Geometry: final body of the model. Coordinates: model frame, mm. A direction names the side the tool comes from. Give positions to 0.01 mm unless a question says otherwise; leave off trailing zeros. Write each loop counter-clockwise with the first axis right and the second up, starting at its lowest first coordinate (ties: lowest second). Pieces come first, ordered by that corner, then holes. Notation, with made-up numbers: M -39.5,-5.75 L -23.5,-5.75 A22 ccw -23.5,7.25 Z; hole C 17.25,69.5 d2. An arc over 180 degrees is marked long. Use a Markdown table: item, result. Add a question column.
(1) Cut plane A-A (z = -4.5). Output: boundary loops of the cut face in (x, y).
(2) Pin query (flat end, axial travel): pin 1 Ø1 at (x, y) = (-1.5, -3.5) entering from -Z; pin 2 Ø1.5 at (y, z) = (-1, -3.5) entering from +X. Return the tip coordinate at first contact, or that it passes through.
(3) Material intervals for L1, parallel to X at y = -3.75, z = 4.75; L2, parallel to Z at x = -1, y = -2.25; L3, parallel to X at y = -3, z = -0.5, sorted ascending.
(4) Draft query along Z for faces 1 (the flat face through (-0.04, -2.99, -6.58)), 2 (the flat face through (0, 0, 0)), 3 (the conical face through (8.223, -1.972, 6.114)), 4 (the conical face through (-1.35, -3.288, 1.375)). Return one class per face: released by +Z, released by -Z, zero draft, split by the parting line, or undercut.
(5) Reachability of faces 5 (the flat face through (0.04, -2.99, 6.58)), 6 (the flat face through (0, -6, -2)), 7 (the conical face through (8.24, -1.97, -6.1)), 8 (the conical face through (-8.24, -1.97, 6.1)), 9 (the conical face through (1.375, -3.288, 1.35)) from +Z, -Z, +X, -X, +Y, -Y: full face, straight path, thin tool, end or side. Return the list, or none.
(6) Cut plane B-B (y = -1.75). State how many separate pieces and enclosed holes the cut face has, plus the area to 3 significant figures.
```python
from build123d import *

# Parameters (mm, degrees)
BOSS_EXTRUDE1_DEPTH = 4
BOSS_EXTRUDE1_DRAFT = 1
SHELL1_T            = -0.5
SKETCH2_R           = 2
BOSS_EXTRUDE2_DEPTH = 5.5
BOSS_EXTRUDE2_TAPER = 1.5
SKETCH4_R           = 1.605977431
CUT_EXTRUDE1_DEPTH  = 5.5
CUT_EXTRUDE1_DRAFT  = 1.5
BOSS_EXTRUDE3_DEPTH = 2.5
BOSS_EXTRUDE4_DEPTH = 2.5


with BuildPart() as part:
    # Sketch1 → Boss-Extrude1 (with draft: the straight prism first)
    with BuildSketch(Plane(origin=(0, 0, 0), x_dir=(1, 0, 0), z_dir=(0, 1, 0))):
        with BuildLine():
            Line((-7.5, -6.375), (7.5, -6.375))
            ThreePointArc((7.5, -6.375), (8.207106781, -6.082106781), (8.5, -5.375))
            Line((8.5, -5.375), (8.5, 5.375))
            ThreePointArc((8.5, 5.375), (8.207106781, 6.082106781), (7.5, 6.375))
            Line((7.5, 6.375), (-7.5, 6.375))
            ThreePointArc((-7.5, 6.375), (-8.207106781, 6.082106781), (-8.5, 5.375))
            Line((-8.5, 5.375), (-8.5, -5.375))
            ThreePointArc((-8.5, -5.375), (-8.207106781, -6.082106781), (-7.5, -6.375))
        make_face()
    extrude(amount=-BOSS_EXTRUDE1_DEPTH)
    # Boss-Extrude1: the draft: its side faces are tilted about the plane it starts from
    boss_extrude1_sides = [part.faces().sort_by_distance(p)[0] for p in [
        (0, -2, 6.375),
        (8.207106781, -2, 6.082106781),
        (8.5, -2, 0),
        (8.207106781, -2, -6.082106781),
        (0, -2, -6.375),
        (-8.207106781, -2, -6.082106781),
        (-8.5, -2, 0),
        (-8.207106781, -2, 6.082106781),
    ]]
    draft(boss_extrude1_sides, Plane(origin=(0, 0, 0), x_dir=(1, 0, 0), z_dir=(0, 1, 0)), BOSS_EXTRUDE1_DRAFT)

    # Shell1
    shell1_openings = [part.faces().sort_by_distance(p)[0] for p in [
        (0, -4, 0),
    ]]
    offset(amount=SHELL1_T, openings=shell1_openings, kind=Kind.INTERSECTION)

    # Sketch2 → Boss-Extrude2 (add)
    with BuildSketch(Plane.XZ.offset(0.5)):
        Circle(SKETCH2_R)
    extrude(amount=BOSS_EXTRUDE2_DEPTH, taper=BOSS_EXTRUDE2_TAPER)

    # Rib1: read off the stored shape, not the designer's step
    # Rib1: loft between two sections, ruled curve by curve
    rib1_from = [
        Edge.make_line((1.982008604, -0.5, 0.267660037), (3, -0.5, 0.25)),
        Edge.make_line((1.982008604, -0.5, -0.267660037), (3, -0.5, -0.25)),
        Edge.make_line((3, -0.5, -0.25), (3, -0.5, 0.25)),
        Edge.make_line((1.982008604, -0.5, -0.267660037), (1.982008604, -0.5, 0.267660037)),
    ]
    rib1_to = [
        Edge.make_line((1.83774048, -6, 0.259542201), (2.387789079, -6, 0.25)),
        Edge.make_line((1.83774048, -6, -0.259542201), (2.387789079, -6, -0.25)),
        Edge.make_line((2.387789079, -6, -0.25), (2.387789079, -6, 0.25)),
        Edge.make_line((1.83774048, -6, -0.259542201), (1.83774048, -6, 0.259542201)),
    ]
    rib1 = Solid(Shell([*[Face.make_surface_from_curves(rib1_from[k], rib1_to[k]) for k in range(4)], Face(Wire(rib1_from)), Face(Wire(rib1_to))]))
    add(rib1)

    # CirPattern1: read off the stored shape, not the designer's step
    # CirPattern1: loft between two sections, ruled curve by curve
    cirpattern1_from = [
        Edge.make_line((-0.267660037, -0.5, 1.982008604), (-0.25, -0.5, 3)),
        Edge.make_line((0.267660037, -0.5, 1.982008604), (0.25, -0.5, 3)),
        Edge.make_line((0.25, -0.5, 3), (-0.25, -0.5, 3)),
        Edge.make_line((0.267660037, -0.5, 1.982008604), (-0.267660037, -0.5, 1.982008604)),
    ]
    cirpattern1_to = [
        Edge.make_line((-0.259542201, -6, 1.83774048), (-0.25, -6, 2.387789079)),
        Edge.make_line((0.259542201, -6, 1.83774048), (0.25, -6, 2.387789079)),
        Edge.make_line((0.25, -6, 2.387789079), (-0.25, -6, 2.387789079)),
        Edge.make_line((0.259542201, -6, 1.83774048), (-0.259542201, -6, 1.83774048)),
    ]
    cirpattern1 = Solid(Shell([*[Face.make_surface_from_curves(cirpattern1_from[k], cirpattern1_to[k]) for k in range(4)], Face(Wire(cirpattern1_from)), Face(Wire(cirpattern1_to))]))
    add(cirpattern1)

    # CirPattern1 2: loft between two sections, ruled curve by curve
    cirpattern1_2_from = [
        Edge.make_line((-1.982008604, -0.5, -0.267660037), (-3, -0.5, -0.25)),
        Edge.make_line((-1.982008604, -0.5, 0.267660037), (-3, -0.5, 0.25)),
        Edge.make_line((-3, -0.5, 0.25), (-3, -0.5, -0.25)),
        Edge.make_line((-1.982008604, -0.5, 0.267660037), (-1.982008604, -0.5, -0.267660037)),
    ]
    cirpattern1_2_to = [
        Edge.make_line((-1.83774048, -6, -0.259542201), (-2.387789079, -6, -0.25)),
        Edge.make_line((-1.83774048, -6, 0.259542201), (-2.387789079, -6, 0.25)),
        Edge.make_line((-2.387789079, -6, 0.25), (-2.387789079, -6, -0.25)),
        Edge.make_line((-1.83774048, -6, 0.259542201), (-1.83774048, -6, -0.259542201)),
    ]
    cirpattern1_2 = Solid(Shell([*[Face.make_surface_from_curves(cirpattern1_2_from[k], cirpattern1_2_to[k]) for k in range(4)], Face(Wire(cirpattern1_2_from)), Face(Wire(cirpattern1_2_to))]))
    add(cirpattern1_2)

    # CirPattern1 3: loft between two sections, ruled curve by curve
    cirpattern1_3_from = [
        Edge.make_line((0.267660037, -0.5, -1.982008604), (0.25, -0.5, -3)),
        Edge.make_line((-0.267660037, -0.5, -1.982008604), (-0.25, -0.5, -3)),
        Edge.make_line((-0.25, -0.5, -3), (0.25, -0.5, -3)),
        Edge.make_line((-0.267660037, -0.5, -1.982008604), (0.267660037, -0.5, -1.982008604)),
    ]
    cirpattern1_3_to = [
        Edge.make_line((0.259542201, -6, -1.83774048), (0.25, -6, -2.387789079)),
        Edge.make_line((-0.259542201, -6, -1.83774048), (-0.25, -6, -2.387789079)),
        Edge.make_line((-0.25, -6, -2.387789079), (0.25, -6, -2.387789079)),
        Edge.make_line((-0.259542201, -6, -1.83774048), (0.259542201, -6, -1.83774048)),
    ]
    cirpattern1_3 = Solid(Shell([*[Face.make_surface_from_curves(cirpattern1_3_from[k], cirpattern1_3_to[k]) for k in range(4)], Face(Wire(cirpattern1_3_from)), Face(Wire(cirpattern1_3_to))]))
    add(cirpattern1_3)


with BuildPart() as cut_extrude1_tool:
    # Sketch4 → Cut-Extrude1 (with draft: the straight prism first)
    with BuildSketch(Plane.XZ.offset(6)):
        Circle(SKETCH4_R)
    extrude(amount=-CUT_EXTRUDE1_DEPTH)
    # Cut-Extrude1: the draft: its side faces are tilted about the plane it starts from
    cut_extrude1_sides = [cut_extrude1_tool.faces().sort_by_distance(p)[0] for p in [
        (-1.605977431, -3.25, 0),
    ]]
    draft(cut_extrude1_sides, Plane.XZ.offset(6), CUT_EXTRUDE1_DRAFT)


with BuildPart() as part_1:
    add(part.part)

    # Cut-Extrude1: cut by cut_extrude1_tool
    add(cut_extrude1_tool.part, mode=Mode.SUBTRACT)

    # Sketch5 → Boss-Extrude3 (add, symmetric)
    with BuildSketch(Plane(origin=(0, 0, 0), x_dir=(0, 0, -1), z_dir=(1, 0, 0))):
        Polygon((6.44482026, -4), (6.40991013, -2), (6.70991013, -2), align=None)
        Polygon((-6.70991013, -2), (-6.44482026, -4), (-6.40991013, -2), align=None)
    extrude(amount=BOSS_EXTRUDE3_DEPTH, both=True)

    # Sketch6 → Boss-Extrude4 (add, symmetric)
    with BuildSketch(Plane.XY):
        Polygon((8.56982026, -4), (8.53491013, -2), (8.83491013, -2), align=None)
        Polygon((-8.83491013, -2), (-8.56982026, -4), (-8.53491013, -2), align=None)
    extrude(amount=BOSS_EXTRUDE4_DEPTH, both=True)


solid = part_1.part
```
Answer list:
| question | item | result |
|---|---|---|
| 1 | outline | M -8.57,-4 L -8.07,-4 L -8.01,-0.5 L 8.01,-0.5 L 8.07,-4 L 8.57,-4 L 8.5,0 L -8.5,0 Z |
| 2 | pin 1 | z = -6.58 |
| 2 | pin 2 | x = 8.53 |
| 3 | L1 | -8.57 to -8.07, 8.07 to 8.57 |
| 3 | L2 | -6.68 to -5.91, -1.68 to -1.38, 1.38 to 1.68, 5.91 to 6.68 |
| 3 | L3 | -8.7 to -8.05, -1.87 to -1.61, 1.61 to 1.87, 8.05 to 8.7 |
| 4 | face 1 | released by -Z |
| 4 | face 2 | zero draft |
| 4 | face 3 | released by +Z |
| 4 | face 4 | undercut |
| 5 | face 5 | +Z, +X, -X, -Y |
| 5 | face 6 | +Z, -Z, +X, -X, -Y |
| 5 | face 7 | -Z, +X, +Y |
| 5 | face 8 | +Z, -X, +Y |
| 5 | face 9 | -Y |
| 6 | separate pieces | 2 |
| 6 | enclosed holes | 2 |
| 6 | area | 33.0 mm² |
